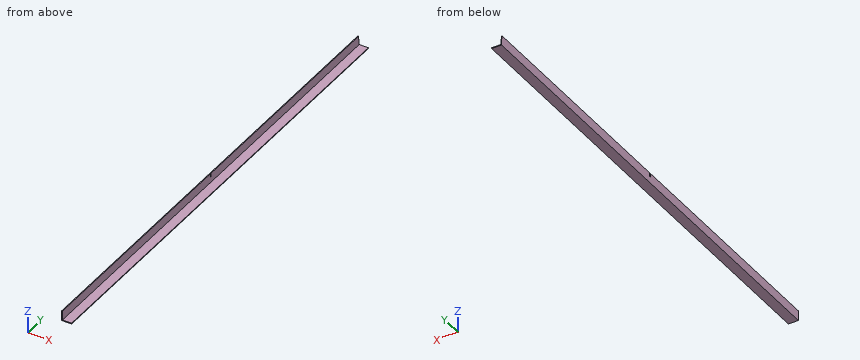
```python
from build123d import *

# Parameters (mm, degrees)
F1_DEPTH = 1835.15
F2_W     = 3.96875
F2_H     = 13.49375
F3_DEPTH = 25.4


with BuildPart() as f1:
    # F0 (on Front) → F1 (new body)
    with BuildSketch(Plane.XZ):
        Polygon((-18.553972, 20.450408), (-21.728972, 20.450408), (-21.728972, -17.649592), (16.371028, -17.649592), (16.371028, -14.474592), (-18.553972, -14.474592), align=None)
    extrude(amount=F1_DEPTH)

    # F2 (on face) → F3 (cut)
    with BuildSketch(Plane(origin=(-21.728972, 0, 0), x_dir=(0, -1, 0), z_dir=(-1, 0, 0))):
        with Locations((917.575, 13.703533)):
            Rectangle(F2_W, F2_H)
        with Locations((1.984375, 13.703533)):
            Rectangle(F2_W, F2_H)
    extrude(amount=-F3_DEPTH, mode=Mode.SUBTRACT)


solid = f1.part
```
Input: part model. Units: mm. Frame: model coordinates. Round coordinates to 2 decimals unless told otherwise and drop trailing zeros. Loops run counter-clockwise (first coordinate to the right, second up) from the corner with the lowest first, then second, coordinate; pieces in that order, holes last. Notation, with made-up numbers: (48, 77.5) -> (59, 77.5) arc R23 ccw to (59, 116.5) -> close; hole circle Ø6 at (-8, 33). An arc over 180 degrees is marked (long way). One line per item, written item: value.
(1) Section B-B (y = -343.5). Return the cut outline in (x, z).
Geometry check:
outline: (-21.73, -17.65) -> (16.37, -17.65) -> (16.37, -14.47) -> (-18.55, -14.47) -> (-18.55, 20.45) -> (-21.73, 20.45) -> close
(2) Material intervals for line 1 (Y direction, x = -19, z = 11); line 2 (X direction, y = -1534, z = 9.5); line 3 (Z direction, x = 13.5, y = -1130), sorted ascending. Write a range as [from, to].
Geometry check:
line 1: [-1835.15, -919.56], [-915.59, -3.97]
line 2: [-21.73, -18.55]
line 3: [-17.65, -14.47]
(3) Section C-C (x = -7). Return the cut outline in (y, z).
Geometry check:
outline: (-1835.15, -17.65) -> (0, -17.65) -> (0, -14.47) -> (-1835.15, -14.47) -> close
(4) Section A-A (z = -1.5). Return the cut outline in (x, y), plus the area to 3 significant figures.
Geometry check:
outline: (-21.73, -1835.15) -> (-18.55, -1835.15) -> (-18.55, 0) -> (-21.73, 0) -> close
area: 5,830 mm2
(5) Pin query (flat end, axial travel): pin 1 (2 mm diameter, centred on y = -1521.5, z = -12.5, fed in from +X); pin 2 (1 mm diameter, centred on x = -20.5, y = -917.5, fed in from +Z); pin 3 (3.5 mm diameter, centred on x = -19.5, z = 17, fed in from +Y); pin 4 (4 mm diameter, centred on x = -15, z = 10.5, fed in from +Y) (3 decimals). Return the tip coordinate at first contact, or that it passes through.
Geometry check:
pin 1: x = -18.55
pin 2: z = 6.96
pin 3: y = -3.97
pin 4: through
